Check sheet for the modelled part. Datum: model origin and axes. Units: mm. Face numbers are marked on the shaded views. A direction names the side the tool comes from. Give positions to 0.01 mm unless a question says otherwise; leave off trailing zeros. Loops run counter-clockwise (first coordinate to the right, second up) from the corner with the lowest first, then second, coordinate; pieces in that order, holes last. Notation, with made-up numbers: M 83.25,-28 L 138.25,-28 A16 cw 138.25,-7 Z; hole C 43,25 d11. An arc over 180 degrees is marked long. Write each question's results on one line, items separated by ' | '. Start each with the question number.
1. Draft check along Y on the marked faces 1, 2, 3 and 4. Enter one of: pulls with the +Y half, pulls with the -Y half, needs draft (parallel to the pull), parting line crosses it, or undercut.
2. Sectioned sample at D-D on y = -7. Record the cut outline in (x, z).
3. Tool access check on the marked faces 5 and 6. Record the directions out of +Z, -Z, +X, -X, +Y, -Y that give a thin tool (end or side, any length) a straight path to the whole face; none if there is none.
4. Sectioned sample at A-A on z = -1.8. Record the cut outline in (x, y), and give its area (3 significant figures).
5. Sectioned sample at C-C on x = 9. Record the cut outline in (y, z).
6. Material ranges on line 1 along X through (y, z) = (8, 0.15); line 2 along Y through (x, z) = (3.5, 0.75); line 3 along X through (y, z) = (-37.5, 0.5), recorded low to high.
7. Sectioned sample at B-B on y = 4. Record the cut outline in (x, z).
8. Go/stop test with flat-tipped pins: pin 1 (2 mm diameter, centred on y = -26, z = -1, fed in from -X); pin 2 (3 mm diameter, centred on y = 3.5, z = 2, fed in from -X). Record where each tip stops, or that it passes through.
```python
from build123d import *

# Parameters (mm, degrees)
SKETCH_1_R      = 5
EXTRUDE_1_DEPTH = 3


with BuildPart() as part:
    # Эскиз1 → Бобышка-Вытянуть1 (new body, symmetric)
    with BuildSketch(Plane.XY):
        with BuildLine():
            Line((4.916234413, -56.120413603), (25.760048074, -2.486528587))
            ThreePointArc((25.760048074, -2.486528587), (28.806805421, -0.347478176), (31.992021255, 1.579350067))
            Line((31.992021255, 1.579350067), (41.693220111, 7.005736507))
            Line((41.693220111, 7.005736507), (38.489887361, 12.920302494))
            Line((38.489887361, 12.920302494), (34.365244293, 10.68639315))
            ThreePointArc((34.365244293, 10.68639315), (33.923481874, 10.203655675), (33.874797711, 9.55110732))
            ThreePointArc((33.874797711, 9.55110732), (31.465191403, 5.552741192), (27.545035778, 8.087600975))
            ThreePointArc((27.545035778, 8.087600975), (27.214853309, 8.652551452), (26.606025774, 8.892381677))
            Line((26.606025774, 8.892381677), (0.41924208, 9.991207939))
            ThreePointArc((0.41924208, 9.991207939), (-8.687811377, 4.951962588), (-8.383148839, -5.451863492))
            ThreePointArc((-8.383148839, -5.451863492), (-0.194512316, -29.232087684), (-4.16010245, -54.068088281))
            ThreePointArc((-4.16010245, -54.068088281), (-5.14748476, -55.852284698), (-6.476272813, -57.39908882))
            ThreePointArc((-6.476272813, -57.39908882), (-6.89807893, -59.725920701), (-4.806109838, -60.82852322))
            ThreePointArc((-4.806109838, -60.82852322), (-0.738045269, -59.854283225), (3.097962953, -58.185950579))
            ThreePointArc((3.097962953, -58.185950579), (4.190313841, -57.314464556), (4.916234413, -56.120413603))
        make_face()
        Circle(SKETCH_1_R, mode=Mode.SUBTRACT)
    extrude(amount=EXTRUDE_1_DEPTH, both=True)


solid = part.part
```
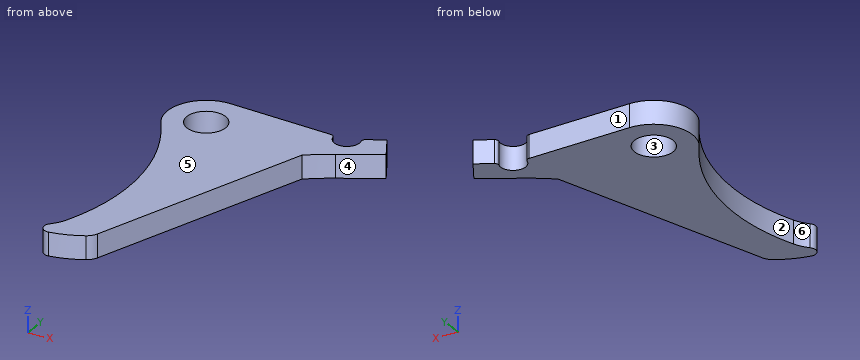
Output values:
1) face 1: pulls with the +Y half | face 2: undercut | face 3: undercut | face 4: pulls with the -Y half
2) outline: M -7.41,-3 L 24.01,-3 L 24.01,3 L -7.41,3 Z
3) face 5: +Z, +X, -X, +Y, -Y | face 6: +Z, -Z, -X
4) outline: M -8.38,-5.45 A51.85 cw -4.16,-54.07 A10 cw -6.48,-57.4 A2 ccw -4.81,-60.83 A23.91 ccw 3.1,-58.19 A4 ccw 4.92,-56.12 L 25.76,-2.49 A54.69 cw 31.99,1.58 L 41.69,7.01 L 38.49,12.92 L 34.37,10.69 A1 ccw 33.87,9.55 A3.25 cw long 27.55,8.09 A1 ccw 26.61,8.89 L 0.42,9.99 A10 ccw Z; hole C 0,0 d10 | area: 1,440 mm2
5) outline: M -45.61,-3 L 9.63,-3 L 9.63,3 L -45.61,3 Z
6) line 1: -6 to 27.56, 33.9 to 41.15 | line 2: -57.94 to -3.57, 3.57 to 9.86 | line 3: -0.14 to 12.15
7) outline: M -9.17,-3 L -3,-3 L -3,3 L -9.17,3 Z; M 3,-3 L 36.32,-3 L 36.32,3 L 3,3 Z
8) pin 1: x = -0.74 | pin 2: x = -9.8
